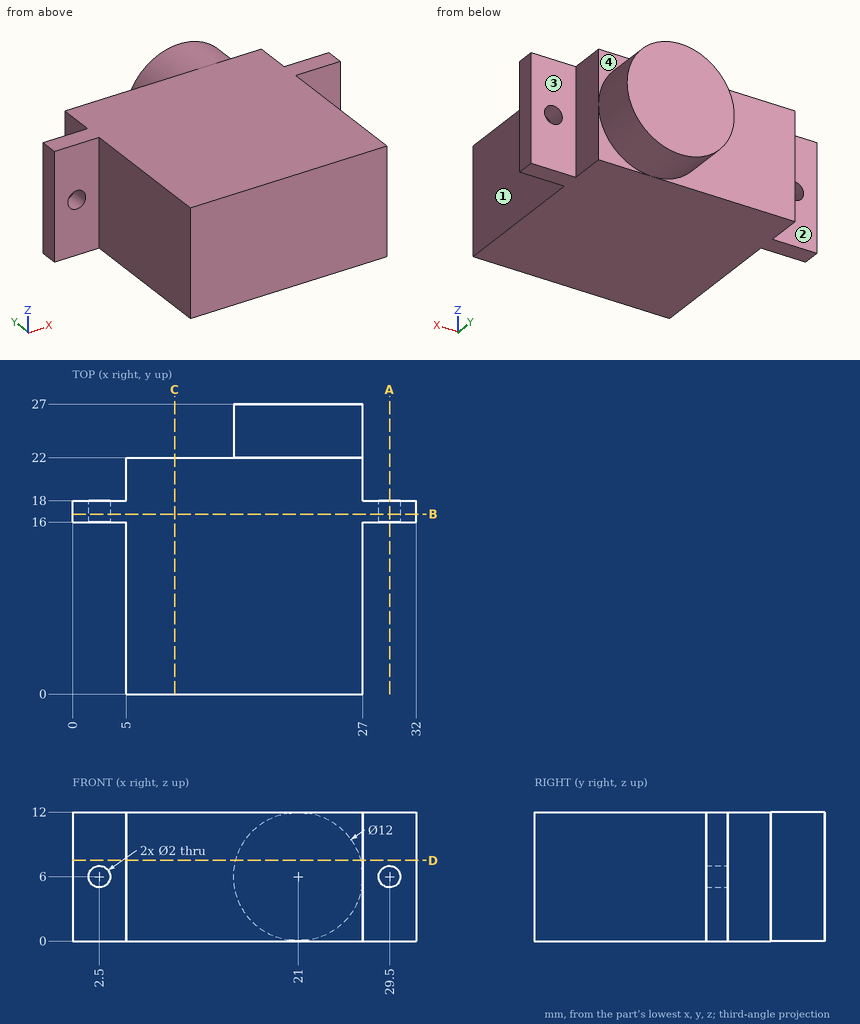
Study the drawing (mm; zero at the part's minimum x, y, z) and answer. A direction names the side the tool comes from. Round coordinates to 2 decimals unless told otherwise and drop trailing zeros. Write each loop counter-clockwise with the first axis right and the second up, starting at its lowest first coordinate (ties: lowest second). Pieces come first, ordered by that corner, then holes.
Q1. A tool of negligible diameter and unlimited length cuts with its end or side. For the marked faces 1, 2, 3 and 4, from which of +Z, -Z, +X, -X, +Y, -Y can it reach the whole face along a straight path? Write none if from no direction.
Values:
face 1: +Z, -Z, +X, -Y
face 2: +Z, -Z, -X, +Y
face 3: +Z, -Z, +X, +Y
face 4: +Z, +X, +Y
Q2. Find section D-D on z = 7.5. Determine the outline of the cut face in (x, y).
Values:
outline: (0, 16) - (5, 16) - (5, 0) - (27, 0) - (27, 16) - (32, 16) - (32, 18) - (27, 18) - (27, 22) - (26.81, 22) - (26.81, 27) - (15.19, 27) - (15.19, 22) - (5, 22) - (5, 18) - (0, 18) - close
Q3. Straight lines are drawn through the part: line 1 (X direction, y = 16.55, z = 6); line 2 (Z direction, x = 29.5, y = 17.05); line 3 (X direction, y = 21.5, z = 1.5). For each, find the intervals that lie inside material, in ascending order.
Values:
line 1: x = 0 to 1.5, 3.5 to 28.5, 30.5 to 32
line 2: z = 0 to 5, 7 to 12
line 3: x = 5 to 27
Q4. Find section B-B on y = 16.75. Determine the outline of the cut face in (x, z).
Values:
outline: (0, 0) - (32, 0) - (32, 12) - (0, 12) - close; hole circle Ø2 at (2.5, 6); hole circle Ø2 at (29.5, 6)
Q5. Find section C-C on x = 9.5. Determine the outline of the cut face in (y, z).
Values:
outline: (0, 0) - (22, 0) - (22, 12) - (0, 12) - close
Q6. Flat-ended cylindrical pins translate along their axes: P1, Ø5, axis at y = 5.5, z = 10.5, coming from the -X side; P2, Ø1.5, axis at x = 3, z = 3.5, coming from the -Y side; P3, Ø6, axis at x = 10.5, z = 3.5, coming from the +Y side; P4, Ø1.8, axis at x = 29.5, z = 6, coming from the -Y side. Find the tip coordinate at first contact, or state that the pin passes through.
Values:
P1: stops at x = 5
P2: stops at y = 16
P3: stops at y = 22
P4: passes through
Q7. Find section A-A on x = 29.5. Determine the outline of the cut face in (y, z), and give its area (3 significant figures).
Values:
outline: (16, 0) - (18, 0) - (18, 5) - (16, 5) - close; (16, 7) - (18, 7) - (18, 12) - (16, 12) - close
area: 20.0 mm2
